The model under review builds one solid part; all positions refer to its coordinate system, in mm. Face numbers are marked on the shaded views. Coordinates: 2 decimals unless noted, no trailing zeros. Order: outer loops, then holes, each group sorted by start corner. A loop starts at its lowest first (then second) coordinate and runs counter-clockwise, first axis right, second up.
from build123d import *

# Parameters (mm, degrees)
SKETCH_R                    = 21
PAD_DEPTH                   = 14
SKETCH001_R                 = 9.05
POCKET_DEPTH                = 4
SKETCH002_R                 = 8.05
POCKET001_DEPTH             = 14.001
SKETCH003_R                 = 15
POCKET002_DEPTH             = 8.001
POCKET003_DEPTH             = 8
SKETCH005_R                 = 3.5
POCKET004_DEPTH             = 8
FILLET_R                    = 2
SKETCH006_R                 = 4
PAD001_DEPTH                = 6
SKETCH007_R                 = 1.65
POCKET005_DEPTH             = 14.001
SKETCH046_R                 = 25
POCKET031_DEPTH             = 6
CHAMFER003068012002052_SIZE = 0.4


with BuildPart() as part:
    # Sketch → Pad (new body)
    with BuildSketch(Plane.XY):
        Circle(SKETCH_R)
    extrude(amount=PAD_DEPTH)

    # Sketch001 (on DatumPlane) → Pocket (cut)
    with BuildSketch(Plane.XY):
        Circle(SKETCH001_R)
    extrude(amount=POCKET_DEPTH, mode=Mode.SUBTRACT)

    # Sketch002 (on DatumPlane) → Pocket001 (cut, through all)
    with BuildSketch(Plane.XY):
        Circle(SKETCH002_R)
    extrude(amount=POCKET001_DEPTH, mode=Mode.SUBTRACT)

    # Sketch003 (on DatumPlane) → Pocket002 (cut, through all)
    with BuildSketch(Plane.XY.offset(6)):
        Circle(SKETCH003_R)
    extrude(amount=POCKET002_DEPTH, mode=Mode.SUBTRACT)

    # Sketch004 (on DatumPlane) → Pocket003 (cut)
    with BuildSketch(Plane.XY.offset(14)):
        Polygon((-10.606602, 10.606602), (0, 10.606602), (0, 21.213203), align=None)
    extrude(amount=-POCKET003_DEPTH, mode=Mode.SUBTRACT)

    # Sketch005 (on DatumPlane) → Pocket004 (cut)
    with BuildSketch(Plane.XY.offset(14)):
        with Locations((0, 18)):
            Circle(SKETCH005_R)
    extrude(amount=-POCKET004_DEPTH, mode=Mode.SUBTRACT)

    # Fillet
    fillet_edges = [part.edges().sort_by_distance(p)[0] for p in [
        (-1.945126, 20.909722, 10),
        (1.945126, 20.909722, 10),
        (1.643223, 14.909722, 10),
    ]]
    fillet(fillet_edges, radius=FILLET_R)

    # Sketch006 (on DatumPlane) → Pad001 (join)
    with BuildSketch(Plane.XY):
        with Locations((0, 18)):
            Circle(SKETCH006_R)
        with Locations((-12.727922, 12.727922)):
            Circle(SKETCH006_R)
        with Locations((12.727922, 12.727922)):
            Circle(SKETCH006_R)
        with Locations((-15.588457, -9)):
            Circle(SKETCH006_R)
        with Locations((15.588457, -9)):
            Circle(SKETCH006_R)
    extrude(amount=PAD001_DEPTH)

    # Sketch007 (on DatumPlane) → Pocket005 (cut, through all)
    with BuildSketch(Plane.XY):
        with Locations((-12.727922, 12.727922)):
            Circle(SKETCH007_R)
        with Locations((12.727922, 12.727922)):
            Circle(SKETCH007_R)
        with Locations((0, 18)):
            Circle(SKETCH007_R)
        with Locations((-15.588457, -9)):
            Circle(SKETCH007_R)
        with Locations((15.588457, -9)):
            Circle(SKETCH007_R)
        with Locations((0, -18)):
            Circle(SKETCH007_R)
    extrude(amount=POCKET005_DEPTH, mode=Mode.SUBTRACT)

    # Sketch046 (on Face5 of Pocket005) → Pocket031 (cut)
    with BuildSketch(Plane(origin=(0, 0, 0), x_dir=(1, 0, 0), z_dir=(0, 0, -1))):
        Circle(SKETCH046_R)
    extrude(amount=-POCKET031_DEPTH, mode=Mode.SUBTRACT)

    # Chamfer003068012002052
    chamfer003068012002052_edges = [part.edges().sort_by_distance(p)[0] for p in [
        (-3.499121, 17.921582, 14),
        (-4.27738, 19.772747, 14),
        (-7.047855, 14.165348, 14),
        (-12.518313, -16.860956, 14),
        (-5.740251, -13.858193, 14),
        (16.860956, 12.518313, 14),
        (12.118742, 8.839462, 14),
        (4.27738, 19.772747, 14),
        (3.402691, 15.295524, 14),
        (3.499491, 18.059668, 14),
        (3.450776, 17.415069, 14),
        (-1.65, -18, 14),
        (-17.238457, -9, 14),
        (13.938457, -9, 14),
        (-14.377922, 12.727922, 14),
        (11.077922, 12.727922, 14),
        (-9.535985, 18.710024, 6),
        (-14.849242, 14.849242, 6),
        (-20.820342, 2.74105, 6),
        (-18.186533, -10.5, 6),
        (0, -21, 6),
        (18.186533, -10.5, 6),
        (20.607252, -4.042422, 6),
        (19.903312, 6.697625, 6),
        (14.849242, 14.849242, 6),
        (9.535985, 18.710024, 6),
        (4.27738, 19.772747, 6),
        (3.499491, 18.059668, 6),
        (3.450776, 17.415069, 6),
        (3.402691, 15.295524, 6),
        (6.75734, 13.391727, 6),
        (10.606602, 10.606602, 6),
        (14.275343, 4.605928, 6),
        (14.75441, -2.703217, 6),
        (12.990381, -7.5, 6),
        (0, -15, 6),
        (-12.990381, -7.5, 6),
        (-14.871673, 1.957893, 6),
        (-11.426085, 9.71826, 6),
        (-7.047855, 14.165348, 6),
        (-3.499121, 17.921582, 6),
        (-4.27738, 19.772747, 6),
        (13.938457, -9, 6),
        (-1.65, -18, 6),
        (-17.238457, -9, 6),
        (11.077922, 12.727922, 6),
        (-14.377922, 12.727922, 6),
    ]]
    chamfer(chamfer003068012002052_edges, length=CHAMFER003068012002052_SIZE)


with BuildPart() as part_1:
    # Body placement: moved
    add(part.part.moved(Location((0, 0, -2))))


solid = part_1.part
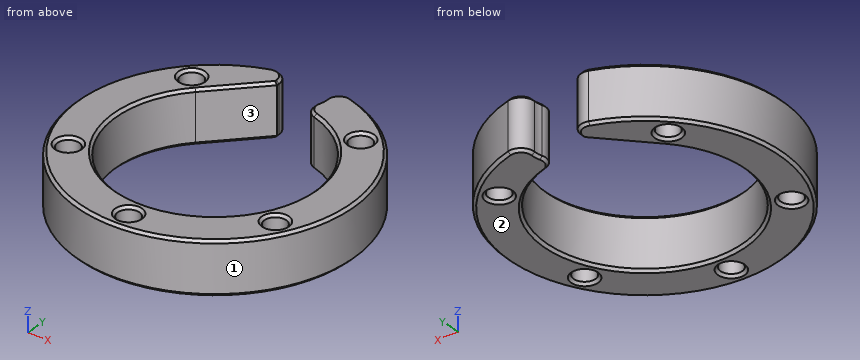
(1) Wall thickness on line 1 (X direction, y = -9.5, z = 9.75); line 2 (X direction, y = 0, z = 10); line 3 (X direction, y = -9, z = 5.25): over which ranges is each line inside the solid? List them lowest first.
(2) The part is to be moulded in two halves that separate along Y. For the marked faces 1, 2 and 3, say which applies: +Y half, -Y half, draft (parallel to the pull), parting line (faces both ways), or undercut.
(3) Insertion check: pin 1 Ø2 at (x, z) = (-15.5, 9) entering from +Y; pin 2 Ø3 at (y, z) = (-7, 8) entering from +X; pin 3 Ø4 at (x, y) = (0, -18) entering from -Z. Each pin has a flat end and moves straight along its axis. Give the tip position at first contact, or say it passes through.
(4) Consider section C-C (z = 5.75). Give the number of separate pieces and of enclosed holes in the cut face, then the cut area to 3 significant figures.
(5) Consider section A-A (y = 0). Give the boundary of the cut face in (x, z), then the cut area to 3 significant figures.
(6) Consider section B-B (x = 0). Give the boundary of the cut face in (y, z), then the cut area to 3 significant figures.
Findings:
1. line 1: x = -18.73 to -17.16, -14.02 to -11.61, 11.61 to 14.02, 17.16 to 18.73
1. line 2: x = -21 to -15, 15 to 21
1. line 3: x = -18.97 to -17.24, -13.94 to -12, 12 to 13.94, 17.24 to 18.97
2. face 1: parting line
2. face 2: draft
2. face 3: undercut
3. pin 1: stops at y = 15.19
3. pin 2: stops at x = 20.27
3. pin 3: stops at z = 4.05
4. separate pieces: 1
4. enclosed holes: 5
4. area: 583 mm2
5. outline: (-21, 4.4) - (-20.6, 4) - (-15.4, 4) - (-15, 4.4) - (-15, 11.6) - (-15.4, 12) - (-20.6, 12) - (-21, 11.6) - close; (15, 4.4) - (15.4, 4) - (20.6, 4) - (21, 4.4) - (21, 11.6) - (20.6, 12) - (15.4, 12) - (15, 11.6) - close
5. area: 95.4 mm2
6. outline: (-21, 4.4) - (-20.6, 4) - (-20.05, 4) - (-19.65, 4.4) - (-19.65, 11.6) - (-20.05, 12) - (-20.6, 12) - (-21, 11.6) - close; (-16.35, 4.4) - (-15.95, 4) - (-15.4, 4) - (-15, 4.4) - (-15, 11.6) - (-15.4, 12) - (-15.95, 12) - (-16.35, 11.6) - close
6. area: 21.0 mm2
